```python
from build123d import *

# Parameters (mm, degrees)
BASE2_DEPTH            = 7.5
MOUNT2_START           = -1.5
MOUNT2_DEPTH           = 3
MOUNT_HOLE2_DEPTH      = 224.418192135
MOUNT_HOLE2_DEPTH_BACK = 224.418192135
SKETCH16_R             = 1.5
SKETCH18_W             = 2.5
SKETCH18_H             = 3
SKETCH19_R             = 1.5
CUT_EXTRUDE10_DEPTH    = 40.784051683


with BuildPart() as part:
    # Sketch13 → base2 (new, symmetric)
    with BuildSketch(Plane(origin=(0, 0, 0), x_dir=(1, 0, 0), z_dir=(0, 1, 0))):
        with BuildLine():
            ThreePointArc((-209.761769634, 10), (-208.70564487, 23.279901188), (-206.809628133, 36.46611731))
            Line((-206.809628133, 36.46611731), (-216.657705663, 38.202599087))
            ThreePointArc((-216.657705663, 38.202599087), (-218.670303662, 24.151569236), (-219.772609758, 10))
            Line((-219.772609758, 10), (-209.761769634, 10))
        make_face()
        with BuildLine():
            ThreePointArc((-209.761769634, -10), (-210, 0), (-209.761769634, 10))
            Line((-209.761769634, 10), (-219.772609758, 10))
            ThreePointArc((-219.772609758, 10), (-220, 0), (-219.772609758, -10))
            Line((-219.772609758, -10), (-209.761769634, -10))
        make_face()
        with BuildLine():
            Line((-216.657705663, -38.202599087), (-206.809628133, -36.46611731))
            ThreePointArc((-206.809628133, -36.46611731), (-208.70564487, -23.279901188), (-209.761769634, -10))
            Line((-209.761769634, -10), (-219.772609758, -10))
            ThreePointArc((-219.772609758, -10), (-218.670303662, -24.151569236), (-216.657705663, -38.202599087))
        make_face()
    extrude(amount=BASE2_DEPTH, both=True)

    # Sketch14 → mount2 (cut)
    with BuildSketch(Plane(origin=(0, 0, 0), x_dir=(1, 0, 0), z_dir=(0, 1, 0)).offset(MOUNT2_START)):
        with BuildLine():
            Line((-209.761769634, -10), (-219.772609758, -10))
            ThreePointArc((-219.772609758, -10), (-218.670303662, -24.151569236), (-216.657705663, -38.202599087))
            Line((-216.657705663, -38.202599087), (-206.809628133, -36.46611731))
            ThreePointArc((-206.809628133, -36.46611731), (-208.70564487, -23.279901188), (-209.761769634, -10))
        make_face()
        with BuildLine():
            Line((-209.761769634, 10), (-219.772609758, 10))
            ThreePointArc((-219.772609758, 10), (-218.670303662, 24.151569236), (-216.657705663, 38.202599087))
            Line((-216.657705663, 38.202599087), (-206.809628133, 36.46611731))
            ThreePointArc((-206.809628133, 36.46611731), (-208.70564487, 23.279901188), (-209.761769634, 10))
        make_face()
    extrude(amount=MOUNT2_DEPTH, mode=Mode.SUBTRACT)

    # Sketch16 → mount hole2 (cut, two sides: drawn at the far end of the back side and taken through both)
    with BuildSketch(Plane(origin=(0, 0, 0), x_dir=(1, 0, 0), z_dir=(0, 1, 0)).offset(-MOUNT_HOLE2_DEPTH_BACK)):
        with Locations(Location((-213.160645195, 28.063131327, 0), (0, 0, 270))):
            Circle(SKETCH16_R)
        with Locations(Location((-214.18186009, 18.738484691, 0), (0, 0, 270))):
            Circle(SKETCH16_R)
        with Locations(Location((-214.18186009, -18.738484691, 0), (0, 0, 270))):
            Circle(SKETCH16_R)
        with Locations(Location((-213.160645195, -28.063131327, 0), (0, 0, 270))):
            Circle(SKETCH16_R)
    extrude(amount=MOUNT_HOLE2_DEPTH + MOUNT_HOLE2_DEPTH_BACK, mode=Mode.SUBTRACT)

    # Sketch18 → bearing (revolve, cut)
    with BuildSketch(Plane(origin=(0, 0, 0), x_dir=(1, 0, 0), z_dir=(0, 1, 0)), mode=Mode.PRIVATE) as bearing_sk:
        with Locations((-215, 1.5)):
            Rectangle(SKETCH18_W, SKETCH18_H)
    revolve(bearing_sk.sketch.rotate(Axis((-215, 0, 0), (1, 0, 0)), 180), axis=Axis((-215, 0, 0), (1, 0, 0)), mode=Mode.SUBTRACT)

    # Sketch19 → Cut-Extrude10 (cut, through all)
    with BuildSketch(Plane(origin=(-215, 0, 0), x_dir=(0, 0, -1), z_dir=(1, 0, 0))):
        Circle(SKETCH19_R)
    extrude(amount=-CUT_EXTRUDE10_DEPTH, mode=Mode.SUBTRACT)


solid = part.part
```
The model under review builds one solid part; all positions refer to its coordinate system, in mm. A direction names the side the tool comes from. Coordinates: 2 decimals unless noted, no trailing zeros. Loops run counter-clockwise (first coordinate to the right, second up) from the corner with the lowest first, then second, coordinate; pieces in that order, holes last. Notation, with made-up numbers: (-5, 74) -> (16, 74) arc R17 cw to (16, 104) -> close; hole circle Ø3 at (85.25, 65). An arc over 180 degrees is marked (long way). Answer as CSV lines item,"result".
Item 1: Take a section at D-D, the plane x = -218.5. State the section outline as (y, z) points, and give its area (3 significant figures).
Results below:
outline,"(-7.5, -25.65) -> (-1.5, -25.65) -> (-1.5, -10) -> (1.5, -10) -> (1.5, -25.65) -> (7.5, -25.65) -> (7.5, 25.65) -> (1.5, 25.65) -> (1.5, 10) -> (-1.5, 10) -> (-1.5, 25.65) -> (-7.5, 25.65) -> close; hole circle Ø3 at (0, 0)"
area,"668 mm2"
Item 2: Take a section at B-B, the plane z = 0. State the section outline as (x, y) points.
Results below:
outline,"(-220, -7.5) -> (-210, -7.5) -> (-210, 7.5) -> (-220, 7.5) -> (-220, 1.5) -> (-216.25, 1.5) -> (-216.25, 3) -> (-213.75, 3) -> (-213.75, -3) -> (-216.25, -3) -> (-216.25, -1.5) -> (-220, -1.5) -> close"
Item 3: Insertion check: pin 1 (0.9 mm diameter, centred on x = -212.5, y = 0.5, fed in from -Z); pin 2 (6 mm diameter, centred on x = -213, y = -3.5, fed in from -Z); pin 3 (3 mm diameter, centred on y = 1.5, z = -24.5, fed in from +X); pin 4 (1.8 mm diameter, centred on x = -214.18, z = -18.74, fed in from +Y). Each pin has a flat end and moves straight along its axis. Give the tip position at first contact, or say it passes through.
Results below:
pin 1,"stops at z = -10"
pin 2,"stops at z = -38.09"
pin 3,"stops at x = -208.38"
pin 4,"passes through"
Item 4: Machinability: for faces 5 (the flat face through (-213, 7.5, -1)), 6 (the flat face through (-213, 1.5, -24)), 7 (the cylindrical face through (-218.1, 0.07, 1.5)), 8 (the cylindrical face through (-214.98, -0.9, 2.86)), 9 (the flat face through (-215, 0, 10)), which of the approach directions +Z, -Z, +X, -X, +Y, -Y give a long, thin tool a straight path to every point of the face, cutting with its end or side? Answer none if there is none.
Results below:
face 5,"+Z, -Z, +X, -X, +Y"
face 6,"-Z, +X, -X"
face 7,"-X"
face 8,"none"
face 9,"+Z, +X, -X"
Item 5: For L1, parallel to Y at x = -209.75, z = 20.5; L2, parallel to X at y = 0.5, z = 2; L3, parallel to Z at x = -212, y = 3.5, list the stretches that pass through material, from the lowest coordinate up.
Results below:
L1,"y = -7.5 to -1.5, 1.5 to 7.5"
L2,"x = -219.99 to -216.25, -213.75 to -209.99"
L3,"z = -37.38 to -29.01, -27.11 to 27.11, 29.01 to 37.38"
Item 6: Take a section at C-C, the plane y = 0. State the section outline as (x, z) points.
Results below:
outline,"(-219.99, -1.5) arc R220 ccw to (-219.77, -10) -> (-209.76, -10) arc R210 cw to (-209.76, 10) -> (-219.77, 10) arc R220 ccw to (-219.99, 1.5) -> (-216.25, 1.5) -> (-216.25, 3) -> (-213.75, 3) -> (-213.75, -3) -> (-216.25, -3) -> (-216.25, -1.5) -> close"
Item 7: Draft analysis for pull direction X (two halves, no side actions). For faces 1 (the flat face through (-213, 1.5, 24)), 2 (the flat face through (-213.75, 0, 0)), 3 (the cylindrical face through (-213.09, 4.46, -29.56)), 4 (the flat face through (-211.66, -4.46, -37.32)), state which applies: +X half, -X half, draft (parallel to the pull), parting line (faces both ways), or undercut.
Results below:
face 1,"draft"
face 2,"undercut"
face 3,"undercut"
face 4,"+X half"
Item 8: Take a section at A-A, the plane z = 11. State the section outline as (x, y) points.
Results below:
outline,"(-219.72, -7.5) -> (-209.71, -7.5) -> (-209.71, -1.5) -> (-219.72, -1.5) -> close; (-219.72, 1.5) -> (-209.71, 1.5) -> (-209.71, 7.5) -> (-219.72, 7.5) -> close"
